Check sheet for the modelled part. Datum: model origin and axes. Units: mm. Round coordinates to 2 decimals unless told otherwise and drop trailing zeros. Loops run counter-clockwise (first coordinate to the right, second up) from the corner with the lowest first, then second, coordinate; pieces in that order, holes last. Notation, with made-up numbers: (4.25, 80.25) -> (45.25, 80.25) arc R19 cw to (45.25, 110.25) -> close; hole circle Ø7 at (-2.75, 42.5). An arc over 180 degrees is marked (long way). One line per item, written item: value. Start each with the question number.
1. Cross-section at A-A on x = 4.5. Record the cut outline in (y, z), then the cut area to 3 significant figures.
2. Go/stop test with flat-tipped pins: pin 1 (1.5 mm diameter, centred on x = 33.5, z = -9, fed in from -Y); pin 2 (0.8 mm diameter, centred on y = 1, z = -68.5, fed in from +X). Record where each tip stops, or that it passes through.
3. Material ranges on L1, parallel to Z at x = 80.5, y = 1; L2, parallel to X at y = 1.1, z = -65; L3, parallel to X at y = 0.35, z = -62, recorded low to high.
4. Cross-section at C-C on x = 80.5. Record the cut outline in (y, z), then the cut area to 3 significant figures.
5. Cross-section at B-B on z = -5. Record the cut outline in (x, y), then the cut area to 3 significant figures.
6. Release check for a two-part mould opening along X. For faces 1 (the face through (-2.357, 0.76, -4.343)), 2 (the face through (39, 1.5, -35)) record: +X half, -X half, draft (parallel to the pull), parting line (faces both ways), or undercut.
7. Cross-section at D-D on y = 1.2. Record the cut outline in (x, z), then the cut area to 3 significant figures.
from build123d import *

# Parameters (mm, degrees)
BOSS_EXTRUDE1_DEPTH  = 1.5
SKETCH3_W            = 4
SKETCH3_H            = 1.5
BOSS_EXTRUDE2_DEPTH  = 3
SKETCH4_R            = 1.08
CUT_EXTRUDE1_DEPTH   = 2.5
LPATTERN1_COUNT      = 2
LPATTERN1_PITCH      = 60
LPATTERN1_COUNT_DIR2 = 2
LPATTERN1_PITCH_DIR2 = 82
LPATTERN2_COUNT      = 2
LPATTERN2_PITCH      = 60
LPATTERN2_COUNT_DIR2 = 2
LPATTERN2_PITCH_DIR2 = 82


with BuildPart() as part:
    # Sketch2 → Boss-Extrude1 (new body)
    with BuildSketch(Plane(origin=(0, 0, 0), x_dir=(1, 0, 0), z_dir=(0, 1, 0))):
        Polygon((0, 0), (79, 0), (79, 70), (0, 70), (0, 50), (15, 50), (15, 30), (0, 30), align=None)
    extrude(amount=BOSS_EXTRUDE1_DEPTH)

    # Sketch3 → Boss-Extrude2 (add)
    with BuildSketch(Plane(origin=(79, 0, 0), x_dir=(0, 0, -1), z_dir=(1, 0, 0))):
        with Locations((5, 0.75)):
            Rectangle(SKETCH3_W, SKETCH3_H)
    boss_extrude2 = extrude(amount=BOSS_EXTRUDE2_DEPTH)

    # Sketch4 → Cut-Extrude1 (cut, through all)
    with BuildSketch(Plane(origin=(0, 1.5, 0), x_dir=(1, 0, 0), z_dir=(0, 1, 0))):
        with Locations((80.5, 5)):
            Circle(SKETCH4_R)
    cut_extrude1 = extrude(amount=-CUT_EXTRUDE1_DEPTH, mode=Mode.SUBTRACT)

    # LPattern1: Boss-Extrude2 2 × 2
    with Locations(*[(-j * LPATTERN1_PITCH_DIR2, 0, -i * LPATTERN1_PITCH) for i in range(LPATTERN1_COUNT) for j in range(LPATTERN1_COUNT_DIR2) if (i, j) != (0, 0)]):
        add(boss_extrude2)

    # LPattern2: Cut-Extrude1 2 × 2
    with Locations(*[(-j * LPATTERN2_PITCH_DIR2, 0, -i * LPATTERN2_PITCH) for i in range(LPATTERN2_COUNT) for j in range(LPATTERN2_COUNT_DIR2) if (i, j) != (0, 0)]):
        add(cut_extrude1, mode=Mode.SUBTRACT)


solid = part.part
Taken from the geometry:
1. outline: (0, -70) -> (1.5, -70) -> (1.5, -50) -> (0, -50) -> close; (0, -30) -> (1.5, -30) -> (1.5, 0) -> (0, 0) -> close
1. area: 75.0 mm2
2. pin 1: stops at y = 0
2. pin 2: stops at x = 79
3. L1: z = -67 to -66.08, -63.92 to -63, -7 to -6.08, -3.92 to -3
3. L2: x = -3 to -2.58, -0.42 to 79.42, 81.58 to 82
3. L3: x = 0 to 79
4. outline: (0, -67) -> (1.5, -67) -> (1.5, -66.08) -> (0, -66.08) -> close; (0, -63.92) -> (1.5, -63.92) -> (1.5, -63) -> (0, -63) -> close; (0, -7) -> (1.5, -7) -> (1.5, -6.08) -> (0, -6.08) -> close; (0, -3.92) -> (1.5, -3.92) -> (1.5, -3) -> (0, -3) -> close
4. area: 5.52 mm2
5. outline: (-3, 0) -> (-2.58, 0) -> (-2.58, 1.5) -> (-3, 1.5) -> close; (-0.42, 0) -> (79.42, 0) -> (79.42, 1.5) -> (-0.42, 1.5) -> close; (81.58, 0) -> (82, 0) -> (82, 1.5) -> (81.58, 1.5) -> close
5. area: 121 mm2
6. face 1: undercut
6. face 2: draft
7. outline: (-3, -67) -> (0, -67) -> (0, -70) -> (79, -70) -> (79, -67) -> (82, -67) -> (82, -63) -> (79, -63) -> (79, -7) -> (82, -7) -> (82, -3) -> (79, -3) -> (79, 0) -> (0, 0) -> (0, -3) -> (-3, -3) -> (-3, -7) -> (0, -7) -> (0, -30) -> (15, -30) -> (15, -50) -> (0, -50) -> (0, -63) -> (-3, -63) -> close; hole circle Ø2.16 at (-1.5, -65); hole circle Ø2.16 at (-1.5, -5); hole circle Ø2.16 at (80.5, -65); hole circle Ø2.16 at (80.5, -5)
7. area: 5,260 mm2
